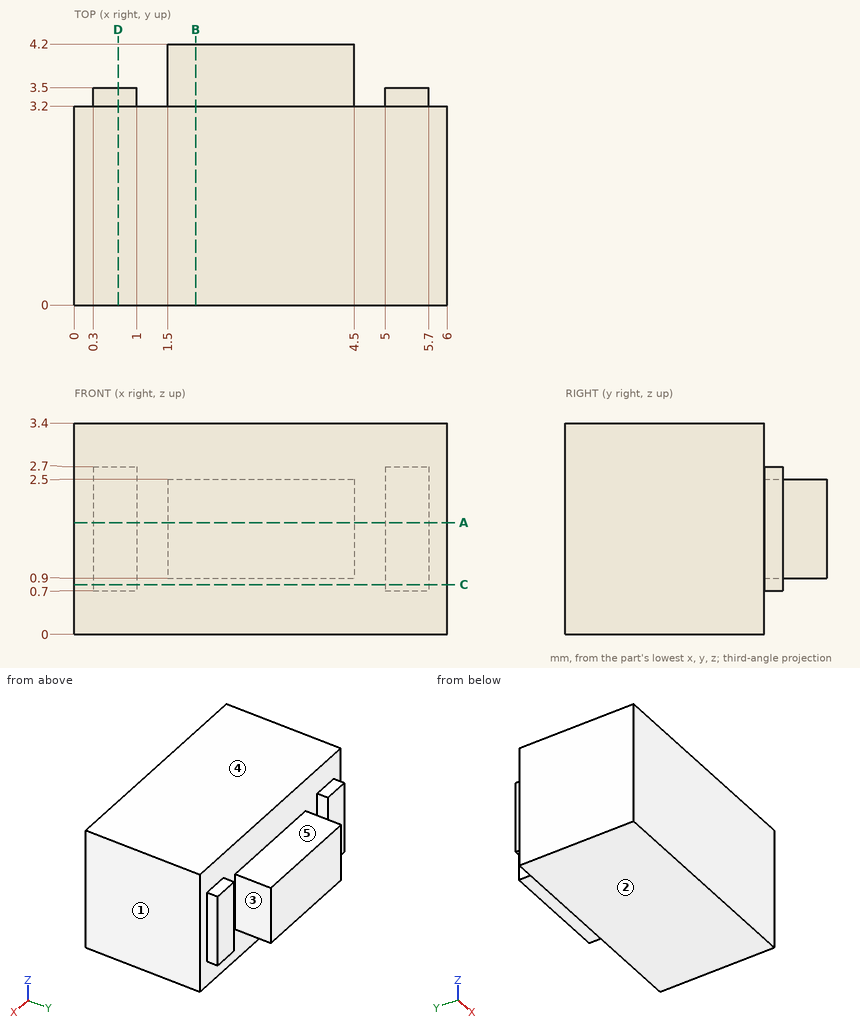
Could you check a few things on this drawing? It's one solid part, dimensions in mm from its lowest x, y, z. A direction names the side the tool comes from. Give positions to 0.01 mm unless a question says otherwise; leave off trailing zeros. Order: outer loops, then holes, each group sorted by start corner. A loop starts at its lowest first (then second) coordinate and runs counter-clockwise, first axis right, second up. Notation, with made-up numbers: M -25.75,-36.75 L 32.25,-36.75 A18 cw 32.25,-29.75 Z; hole C 49.25,-3.75 d5. An arc over 180 degrees is marked long. Use one line per item in the form item = value. Start each with the question number.
Item 1: If we section it at D-D (x = 0.7): Write out the boundary of the cut face in (y, z).
Item 2: We'd pull the mould along X, two halves only. Please class the marked faces 1, 2 and 3: +X half, -X half, draft (parallel to the pull), parting line (faces both ways), or undercut.
Item 3: If I drill on line 1 along X through (y, z) = (3.4, 2.3); line 2 along Y through (x, z) = (0.75, 3); line 3 along Y through (x, z) = (5.05, 1.25), over which ranges is the centre line in solid material (lowest first)?
Item 4: Will these pins go through, and if not, where does the flat tip stop? pin 1 Ø0.8 at (x, y) = (2.5, 4) entering from +Z; pin 2 Ø0.6 at (x, z) = (1, 1.5) entering from +Y; pin 3 Ø0.5 at (y, z) = (4, 2) entering from +X.
Item 5: If we section it at C-C (z = 0.8): Write out the boundary of the cut face in (x, y).
Item 6: If we section it at A-A (z = 1.8): Write out the boundary of the cut face in (x, y), then the cut area to 3 significant figures.
Item 7: If we section it at B-B (x = 1.95): Write out the boundary of the cut face in (y, z), then the cut area to 3 significant figures.
Item 8: For the marked faces 4 and 5, which set-ups out of +Z, -Z, +X, -X, +Y, -Y let a thin tool reach every point of the face, with its end or its side?
Outcome:
q1.outline = M 0,0 L 3.2,0 L 3.2,0.7 L 3.5,0.7 L 3.5,2.7 L 3.2,2.7 L 3.2,3.4 L 0,3.4 Z
q2.face_1 = +X half
q2.face_2 = draft
q2.face_3 = undercut
q3.line_1 = 0.3 to 1, 1.5 to 4.5, 5 to 5.7
q3.line_2 = 0 to 3.2
q3.line_3 = 0 to 3.5
q4.pin_1 = 2.5
q4.pin_2 = 3.5
q4.pin_3 = 4.5
q5.outline = M 0,0 L 6,0 L 6,3.2 L 5.7,3.2 L 5.7,3.5 L 5,3.5 L 5,3.2 L 1,3.2 L 1,3.5 L 0.3,3.5 L 0.3,3.2 L 0,3.2 Z
q6.outline = M 0,0 L 6,0 L 6,3.2 L 5.7,3.2 L 5.7,3.5 L 5,3.5 L 5,3.2 L 4.5,3.2 L 4.5,4.2 L 1.5,4.2 L 1.5,3.2 L 1,3.2 L 1,3.5 L 0.3,3.5 L 0.3,3.2 L 0,3.2 Z
q6.area = 22.6 mm2
q7.outline = M 0,0 L 3.2,0 L 3.2,0.9 L 4.2,0.9 L 4.2,2.5 L 3.2,2.5 L 3.2,3.4 L 0,3.4 Z
q7.area = 12.5 mm2
q8.face_4 = +Z, +X, -X, +Y, -Y
q8.face_5 = +Z, +Y
